Autodesk Inventor part; units mm, degrees
ref_plane "Work Plane1" through (0, 0, -12.6008) normal (0.866, -0.5, 0) x (0, 0, 1)
ref_plane "YZ Plane" through (0, 0, 0) normal (1, 0, 0) x (0, 1, 0)
ref_plane "XZ Plane" through (0, 0, 0) normal (0, 1, 0) x (-1, 0, 0)
sketch "Sketch2" plane through (0, 0, 0) normal (0, 0, 1) x (1, 0, 0)
  line L0 (2.3813, 1.3748) -> (2.3812, -1.3748)
  line L1 (2.3812, -1.3748) -> (0, -2.7496)
  line L2 (0, -2.7496) -> (-2.3812, -1.3748)
  line L3 (-2.3812, 1.3748) -> (-2.3812, -1.3748)
  line L4 (-2.3812, 1.3748) -> (0, 2.7496)
  line L5 (0, 2.7496) -> (2.3813, 1.3748)
  circle A0 centre (0, 0) radius 2.7496 construction
  line L6 (0, 25.4) -> (0, -25.4) construction
  dimension "d3" = 4.7625
extrude "Hexagon1" add sketch "Sketch2" against normal blind 7.9375
sketch "Sketch3" plane through (0, 0, -7.9375) normal (0, 0, -1) x (-1, 0, 0)
  circle A0 centre (0, 0) radius 1.0795
  dimension "d11" = 2.159
sketch "Sketch4" plane through (0, 0, 0) normal (0, 0, 1) x (1, 0, 0)
  point P0 (0, 0)
hole "Hole1" at (0, 0, 0) direction (0, 0, -1) diameter 2.159 depth 6.35 tip angle 118
extrude "Extrusion2" add sketch "Sketch3" along normal blind 4.7625
chamfer "Chamfer1" distance 0.1984 angle 45 1 edges at (1.0795, 0, -12.7)
chamfer "Chamfer2" distance 0.1984 angle 45 1 edges at (0, 1.0795, 0)
thread "Thread1"
ref_plane "Work Plane1" through (0, 0, -12.6008) normal (0.866, -0.5, 0) x (0, 0, 1)
sketch "Sketch5" plane through (0, 0, -12.6008) normal (0.866, -0.5, 0) x (0, 0, 1)
  line L0 (4.6633, 0) -> (4.6633, -2.3812)
  line L1 (4.6633, -1.0795) -> (0.0992, -1.0795)
  line L2 (4.6633, -1.0795) -> (4.3763, -1.0795)
  line L3 (4.3763, -1.0795) -> (4.3763, -0.8769)
  line L4 (4.3763, -0.8769) -> (4.6633, -0.8769)
  line L5 (4.6633, -0.8769) -> (4.6633, -1.0795)
  line L6 (-2.6392, 0) -> (15.1408, 0)
revolve "Revolution1" cut sketch "Sketch5" angle 360 about axis through (0, 0, -10) along (0, 0, 1)
chamfer "Chamfer3" distance 0.1984 angle 45 1 edges at (1.0795, 0, -8.2244)
properties part number "219-1048" material "Steel, Mild"
CAD build for the part. Positions are in the model's coordinates, mm. A direction names the side the tool comes from. Round coordinates to 2 decimals unless told otherwise and drop trailing zeros. Write each loop counter-clockwise with the first axis right and the second up, starting at its lowest first coordinate (ties: lowest second). Pieces come first, ordered by that corner, then holes.
(1) Slice it at C-C, the plane x = -1.8. Write the cut outline in (y, z), and give its area (3 significant figures).
(2) Slice it at B-B, the plane z = -11.5. Write the cut outline in (x, y), and give its area (3 significant figures).
(3) Drop flat-ended pins along their axis: P1, Ø0.5, axis at x = 0.5, y = 0, coming from the +Z side; P2, Ø1, axis at x = -1, z = -10.5, coming from the +Y side. Give the stop position or say it passes through.
(4) 3-axis set-ups, long thin cutter, end or side, ignore diameter. For faces 1 (the face through (-1.07, 0.14, -3.32)), 2 (the face through (0.14, -1.07, -10.43)), 3 (the face through (1.21, -2.05, -3.91)): which of +Z, -Z, +X, -X, +Y, -Y reach the whole face in a straight line?
(5) Probe line 1 along X through (y, z) = (0, -3.25); line 2 along Y through (x, z) = (0.1, -2.25); line 3 along Z through (x, y) = (-0.35, 1.45). List the from-to ranges inside material, lowest first.
(6) Slice it at A-A, the plane z = -5.75. Write the cut outline in (x, y), and give its area (3 significant figures).
From the geometry:
1. outline: (-1.71, -7.94) - (1.71, -7.94) - (1.71, 0) - (-1.71, 0) - close
1. area: 27.2 mm2
2. outline: circle Ø2.16 at (0, 0)
2. area: 3.66 mm2
3. P1: stops at z = -6.55
3. P2: stops at y = 0.96
4. face 1: +Z
4. face 2: -Z
4. face 3: +Z, -Z, +X, -Y
5. line 1: x = -2.38 to -1.08, 1.08 to 2.38
5. line 2: y = -2.69 to -1.07, 1.07 to 2.69
5. line 3: z = -7.94 to 0
6. outline: (-2.38, -1.37) - (0, -2.75) - (2.38, -1.37) - (2.38, 1.37) - (0, 2.75) - (-2.38, 1.37) - close; hole circle Ø2.16 at (0, 0)
6. area: 16.0 mm2
